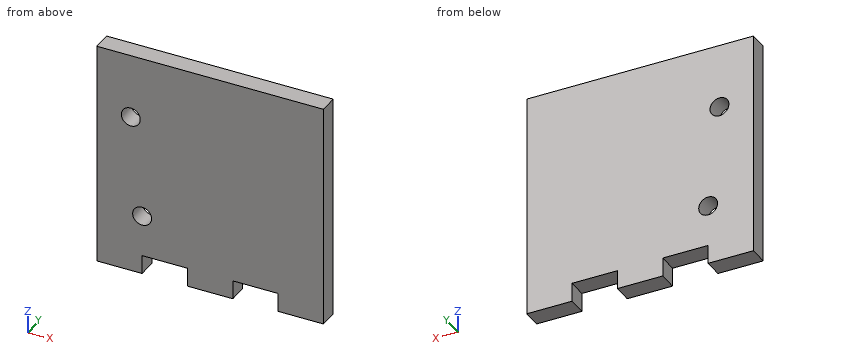
```python
from build123d import *

# Parameters (mm, degrees)
F0_W     = 38.1
F0_H     = 38.1
F1_DEPTH = 3.175
F2_W     = 7.62
F2_H     = 3.175
F2_R     = 1.5875
F3_DEPTH = 3.175
F4_DEPTH = 2.54


with BuildPart() as f1:
    # F0 (on Front) → F1 (new body)
    with BuildSketch(Plane.XZ):
        with Locations((-6.205209, -2.285485)):
            Rectangle(F0_W, F0_H)
    extrude(amount=F1_DEPTH)

    # F2 (on face) → F3 (cut)
    with BuildSketch(Plane.XZ.offset(3.175)):
        with Locations((-13.825209, -19.747985)):
            Rectangle(F2_W, F2_H)
        with Locations((1.414791, -19.747985)):
            Rectangle(F2_W, F2_H)
        with Locations((-19.535628, 5.882839)):
            Circle(F2_R)
        with Locations((-17.635209, -11.156511)):
            Circle(F2_R)
    extrude(amount=-F3_DEPTH, mode=Mode.SUBTRACT)

    # F2 (on face) → F4 (cut)
    with BuildSketch(Plane.XZ.offset(3.175)):
        with Locations((-17.635209, -11.156511)):
            Circle(F2_R)
        with Locations((-19.535628, 5.882839)):
            Circle(F2_R)
    extrude(amount=-F4_DEPTH, mode=Mode.SUBTRACT)


solid = f1.part
```
Geometry check sheet. Reference: the model listing, model coordinates, mm. Round coordinates to 2 decimals unless told otherwise and drop trailing zeros. Order: outer loops, then holes, each group sorted by start corner. A loop starts at its lowest first (then second) coordinate and runs counter-clockwise, first axis right, second up. Notation, with made-up numbers: M 88,-12.75 L 147,-12.75 A27 ccw 147,12.25 Z; hole C 28.5,70.25 d10. An arc over 180 degrees is marked long. Write item = value, one per line.
Q1. Scan line: line 1 (Z direction, x = -2, y = -2.05). Record every from-to range of solid material in increasing order.
Answer block:
line_1 = -18.16 to 16.76
Q2. Section check A-A (y = -2.45). Enter the section's corners in (x, z) (1 decimal).
Answer block:
outline = M -25.3,-21.3 L -17.6,-21.3 L -17.6,-18.2 L -10,-18.2 L -10,-21.3 L -2.4,-21.3 L -2.4,-18.2 L 5.2,-18.2 L 5.2,-21.3 L 12.8,-21.3 L 12.8,16.8 L -25.3,16.8 Z; hole C -19.5,5.9 d3.2; hole C -17.6,-11.2 d3.2
Q3. Depth check by flat-ended pin: pin 1 Ø1.6 at (x, y) = (2.5, -1) entering from -Z. Enter the tip coordinate at first touch or a pass-through.
Answer block:
pin_1 = -18.16
Q4. Section check B-B (x = -20.5). Enter the section's corners in (y, z) (3 decimals), plus the area to 3 significant figures.
Answer block:
outline = M -3.175,-21.335 L 0,-21.335 L 0,4.622 L -3.175,4.622 Z; M -3.175,7.144 L 0,7.144 L 0,16.765 L -3.175,16.765 Z
area = 113 mm^2
Q5. Section check C-C (x = -11). Enter the section's corners in (y, z) (3 decimals).
Answer block:
outline = M -3.175,-18.16 L 0,-18.16 L 0,16.765 L -3.175,16.765 Z
